Part model, mm, in its own coordinate system. A direction names the side the tool comes from. Give positions to 0.01 mm unless a question says otherwise; leave off trailing zeros. Order: outer loops, then holes, each group sorted by start corner. A loop starts at its lowest first (then second) coordinate and runs counter-clockwise, first axis right, second up. Notation, with made-up numbers: (10, -28.5) -> (49, -28.5) arc R24 cw to (49, -2.5) -> close; hole circle Ø10 at (-19.5, -33). An arc over 180 degrees is marked (long way). Write item = value, one per line. Start each with the question number.
(1) Flat gauge pins, fed straight in: pin 1 (3 mm diameter, centred on x = 15, z = 2.5, fed in from +Y); pin 2 (4 mm diameter, centred on x = 0, y = 12.45, fed in from -Z); pin 3 (2.5 mm diameter, centred on x = -7.5, z = 3, fed in from +Y); pin 4 (1.5 mm diameter, centred on x = 0, z = 1.5, fed in from -Y). Where does each tip first touch, or does it go through?
(2) Saw through at A-A, the plane y = 0. List the corners of the cut face in (x, z).
(3) Saw through at C-C, the plane x = 7. List the corners of the cut face in (y, z), then the cut area to 3 significant figures.
(4) Probe line 1 along Y through (x, z) = (0, 1.55); line 2 along X through (y, z) = (-4, 1.25); line 3 along Y through (x, z) = (-8.5, 0.95). List the from-to ranges inside material, lowest first. Write a range as from..to.
(5) Saw through at D-D, the plane z = 2.65. List the corners of the cut face in (x, y) (3 decimals), then the cut area to 3 significant figures.
(6) Saw through at B-B, the plane x = 0. List the corners of the cut face in (y, z), then the cut area to 3 significant figures.
(7) Which spindle directions (+Z, -Z, +X, -X, +Y, -Y) get a long thin tool onto all of the face, cutting with end or side? Do faces 4 (the flat face through (0, -5, 5)), 5 (the flat face through (-10, 2, 2)). Say none if no direction does.
(8) Two-plate mould, pull along X, no slides. Class faces 1 (the flat face through (6, -1.5, 2)), 2 (the cylindrical face through (-4.785, -21.547, 2.465)), 3 (the flat face through (0, -5, 0)): pulls with the +X half, pulls with the -X half, needs draft (parallel to the pull), parting line crosses it, or undercut.
from build123d import *

# Parameters (mm, degrees)
SKETCH_1_R      = 22.071639064
SKETCH_1_R_2    = 2.5
EXTRUDE_1_DEPTH = 5


with BuildPart() as part:
    # 스케치1 → 보스-돌출1 (new body)
    with BuildSketch(Plane.XY):
        Circle(SKETCH_1_R)
        with Locations((0, 12.45)):
            Circle(SKETCH_1_R_2, mode=Mode.SUBTRACT)
        with Locations((-10.782016277, -6.225)):
            Circle(SKETCH_1_R_2, mode=Mode.SUBTRACT)
        with Locations((10.782016277, -6.225)):
            Circle(SKETCH_1_R_2, mode=Mode.SUBTRACT)
        with BuildLine():
            Line((10, 5.5), (10, -1.5))
            Line((10, -1.5), (2.598076211, -1.5))
            ThreePointArc((2.598076211, -1.5), (0, -3), (-2.598076211, -1.5))
            Line((-2.598076211, -1.5), (-10, -1.5))
            Line((-10, -1.5), (-10, 5.5))
            Line((-10, 5.5), (10, 5.5))
        make_face(mode=Mode.SUBTRACT)
    extrude(amount=EXTRUDE_1_DEPTH)


solid = part.part
Results list:
q1.pin_1 = 17.46
q1.pin_2 = through
q1.pin_3 = 21.17
q1.pin_4 = -22.07
q2.outline = (-22.07, 0) -> (-10, 0) -> (-10, 5) -> (-22.07, 5) -> close; (10, 0) -> (22.07, 0) -> (22.07, 5) -> (10, 5) -> close
q3.outline = (-20.93, 0) -> (-1.5, 0) -> (-1.5, 5) -> (-20.93, 5) -> close; (5.5, 0) -> (20.93, 0) -> (20.93, 5) -> (5.5, 5) -> close
q3.area = 174 mm^2
q4.line_1 = -22.07..-3, 5.5..9.95, 14.95..22.07
q4.line_2 = -21.71..-11.92, -9.64..9.64, 11.92..21.71
q4.line_3 = -20.37..-7.25, -5.2..-1.5, 5.5..20.37
q5.outline = circle Ø44.143 at (0, 0); hole circle Ø5 at (-10.782, -6.225); hole (-10, -1.5) -> (-2.598, -1.5) arc R3 ccw to (2.598, -1.5) -> (10, -1.5) -> (10, 5.5) -> (-10, 5.5) -> close; hole circle Ø5 at (0, 12.45); hole circle Ø5 at (10.782, -6.225)
q5.area = 1,330 mm^2
q6.outline = (-22.07, 0) -> (-3, 0) -> (-3, 5) -> (-22.07, 5) -> close; (5.5, 0) -> (9.95, 0) -> (9.95, 5) -> (5.5, 5) -> close; (14.95, 0) -> (22.07, 0) -> (22.07, 5) -> (14.95, 5) -> close
q6.area = 153 mm^2
q7.face_4 = +Z, +X, -X, +Y, -Y
q7.face_5 = +Z, -Z
q8.face_1 = undercut
q8.face_2 = parting line crosses it
q8.face_3 = needs draft
